CAD build for the part. Positions are in the model's coordinates, mm. Face numbers are marked on the shaded views. A direction names the side the tool comes from. Round coordinates to 2 decimals unless told otherwise and drop trailing zeros. Loops run counter-clockwise (first coordinate to the right, second up) from the corner with the lowest first, then second, coordinate; pieces in that order, holes last. Notation, with made-up numbers: (47.5, 45) -> (86.5, 45) arc R26 cw to (86.5, 66) -> close; hole circle Ø6 at (-4.75, 83.25). An arc over 180 degrees is marked (long way). Answer as CSV lines item,"result".
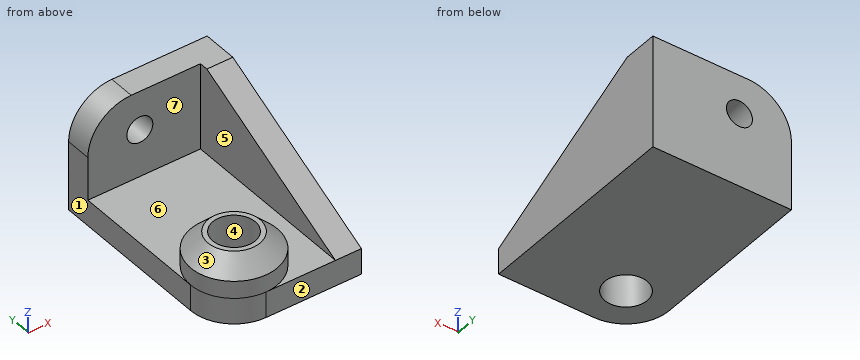
```python
from build123d import *

# Parameters (mm, degrees)
F0_W     = 16
F0_H     = 24
F1_DEPTH = 13
F2_T     = -3
F3_R     = 5
F4_DEPTH = 4
F5_D     = 4.9
F6_SIZE2 = 10
F6_SIZE  = 20
F7_R     = 5
F8_SIZE  = 2
F10_D    = 3
F11_R    = 4.9999


# Not quite as in the source:
# - a fillet or chamfer is up to 0.001 mm smaller than in the source, because OpenCascade refuses the exact size


with BuildPart() as f1:
    # F0 (on Top) → F1 (new body)
    with BuildSketch(Plane.XY):
        with Locations((8, 12)):
            Rectangle(F0_W, F0_H)
    extrude(amount=F1_DEPTH)

    # F2
    f2_openings = [f1.faces().sort_by_distance(p)[0] for p in [
        (8, 0, 6.5),
        (0, 12, 6.5),
        (8, 12, 13),
    ]]
    offset(amount=F2_T, openings=f2_openings)

    # F3 (on face) → F4 (join)
    with BuildSketch(Plane.XY.offset(3)):
        with Locations((5, 5)):
            Circle(F3_R)
    extrude(amount=F4_DEPTH)

    # F5 (through all)
    with Locations(Plane(origin=(0, 0, 0), x_dir=(1, 0, 0), z_dir=(0, 0, -1))):
        with Locations((5, -5)):
            Hole(F5_D / 2)

    # F6
    f6_edges = [f1.edges().sort_by_distance(p)[0] for p in [
        (14.5, 0, 13),
    ]]
    f6_side = f1.faces().sort_by_distance((8, 23.711556, 13))[0]
    chamfer(f6_edges, length=F6_SIZE, length2=F6_SIZE2, reference=f6_side)

    # F7
    f7_edges = [f1.edges().sort_by_distance(p)[0] for p in [
        (0, 22.5, 13),
    ]]
    fillet(f7_edges, radius=F7_R)

    # F8
    f8_edges = [f1.edges().sort_by_distance(p)[0] for p in [
        (0, 5, 7),
    ]]
    chamfer(f8_edges, length=F8_SIZE)

    # F10 (through all)
    with Locations(Plane(origin=(0, 24, 0), x_dir=(-1, 0, 0), z_dir=(0, 1, 0))):
        with Locations((-6, 8.5)):
            Hole(F10_D / 2)

    # F11 (radius 5 in the source; OpenCascade refuses exactly that, so slightly less here)
    f11_edges = [f1.edges().sort_by_distance(p)[0] for p in [
        (0, 0, 1.5),
    ]]
    fillet(f11_edges, radius=F11_R)


solid = f1.part
```
Q1. Probe L1, parallel to Y at x = 5, z = 4.5; L2, parallel to Y at x = 5, z = 5.25; L3, parallel to Z at x = 6, y = 21.7. List the from-to ranges inside material, lowest first. Write a range as [from, to].
Results:
L1,"[0, 2.55], [7.45, 10], [21, 24]"
L2,"[0.25, 2.55], [7.45, 9.75], [21, 24]"
L3,"[0, 7], [10, 13]"
Q2. Drop flat-ended pins along their axis: pin 1 Ø4.5 at (x, y) = (5, 5) entering from +Z; pin 2 Ø1 at (x, z) = (6.5, 6.5) entering from -Y; pin 3 Ø2.5 at (x, y) = (1.5, 2) entering from +Z; pin 4 Ø2 at (x, y) = (7, 5) entering from +Z. Give the stop position or say it passes through.
Results:
pin 1,"through"
pin 2,"y = 1.26"
pin 3,"z = 6.64"
pin 4,"z = 7"
Q3. Tool access for the marked faces 5, 6 and 7: list every direction of +Z, -Z, +X, -X, +Y, -Y with a clear straight run to the whole face (end or side of a thin tool).
Results:
face 5,"+Z, -Y"
face 6,"+Z"
face 7,"+Z, -X"
Q4. Two-plate mould, pull along Y, no slides. Class the marked faces 1, 2, 3 and 4: pulls with the +Y half, pulls with the -Y half, needs draft (parallel to the pull), parting line crosses it, or undercut.
Results:
face 1,"needs draft"
face 2,"pulls with the -Y half"
face 3,"undercut"
face 4,"undercut"
Q5. Slice it at A-A, the plane y = 22.25. Give the cut face in (x, z).
Results:
outline,"(0, 0) -> (16, 0) -> (16, 13) -> (5, 13) arc R5 ccw to (0, 8) -> close; hole circle Ø3 at (6, 8.5)"
Q6. Slice it at C-C, the plane x = 12.5. Give the cut face in (y, z), and give its area (3 significant figures).
Results:
outline,"(0, 0) -> (24, 0) -> (24, 13) -> (21, 13) -> (21, 3) -> (0, 3) -> close"
area,"102 mm2"
Q7. Slice it at D-D, the plane x = 6. Count the separate pieces of the cut face and the enclosed holes in it, and give its area (3 significant figures).
Results:
separate pieces,"3"
enclosed holes,"0"
area,"96.8 mm2"
Q8. Slice it at B-B, the plane z = 2.5. Give the cut face in (x, y).
Results:
outline,"(0, 5) arc R5 ccw to (5, 0) -> (16, 0) -> (16, 24) -> (0, 24) -> close; hole circle Ø4.9 at (5, 5)"
